Check sheet for the modelled part. Datum: model origin and axes. Units: mm. Round coordinates to 2 decimals unless told otherwise and drop trailing zeros. Write each loop counter-clockwise with the first axis right and the second up, starting at its lowest first coordinate (ties: lowest second). Pieces come first, ordered by that corner, then holes.
Item 1: Section check A-A, the plane x = 104. Record the cut outline in (y, z) (3 decimals), plus the area to 3 significant figures.
Item 2: Material ranges on line 1 along Y through (x, z) = (228.5, 7.25) (3 decimals); line 2 along Z through (x, y) = (-241.3, -2.65), recorded low to high.
Item 3: Release check for a two-part mould opening along Y. For faces 1 (the flat face through (4, 0, 5.556)), 2 (the flat face through (4, -5.556, 0)), 3 (the flat face through (4, 0, -5.556)), 4 (the flat face through (4, 5.556, 0)) record: pulls with the +Y half, pulls with the -Y half, needs draft (parallel to the pull), parting line crosses it, or undercut.
Item 4: Depth check by flat-ended pin: pin 1 (5.5 mm diameter, centred on x = -12.7, y = 0, fed in from +Z); pin 2 (6.5 mm diameter, centred on x = 63.5, z = 0, fed in from +Y). Enter the tip coordinate at first touch or a pass-through.
from build123d import *

# Parameters (mm, degrees)
SKETCH1_W             = 19.05
SKETCH1_H             = 19.05
BOSS_EXTRUDE1_DEPTH   = 254
SKETCH3_W             = 2.4892
SKETCH3_H             = 19.05
SKETCH3_AT_POINT_2_W  = 2.4892
SKETCH3_AT_POINT_2_H  = 19.05
LPATTERN1_START       = -11
LPATTERN1_OUTLINE_R   = 2.4892
LPATTERN1_DEPTH       = 22
LPATTERN1_2_OUTLINE_R = 2.4892
LPATTERN1_2_DEPTH     = 22
SKETCH4_W             = 3.96875
SKETCH4_H             = 7.9375
SKETCH4_W_2           = 7.9375
SKETCH4_H_2           = 3.96875
CUT_EXTRUDE1_DEPTH    = 509.178562368


with BuildPart() as part:
    # Sketch1 → Boss-Extrude1 (new, symmetric)
    with BuildSketch(Plane(origin=(0, 0, 0), x_dir=(0, 0, -1), z_dir=(1, 0, 0))):
        Rectangle(SKETCH1_W, SKETCH1_H)
    extrude(amount=BOSS_EXTRUDE1_DEPTH, both=True)

    # Sketch3 → #9 (0.196) Diameter Hole1 (revolve, cut)
    with BuildSketch(Plane(origin=(241.3, 9.525, 0), x_dir=(0, 0, 1), z_dir=(1, 0, 0))):
        with Locations((1.2446, 9.525)):
            Rectangle(SKETCH3_W, SKETCH3_H)
    revolve(axis=Axis((241.3, 15.875, 0), (0, -1, 0)), mode=Mode.SUBTRACT)

    # Sketch3 at point 2 (carried to point 2, square into its face) → #9 (0.196) Diameter Hole1 at 2 (revolve, cut)
    with BuildSketch(Plane(origin=(241.3, 0, 9.525), x_dir=(0, -1, 0), z_dir=(1, 0, 0))):
        with Locations((1.2446, 9.525)):
            Rectangle(SKETCH3_AT_POINT_2_W, SKETCH3_AT_POINT_2_H)
    revolve(axis=Axis((241.3, 0, 15.875), (0, 0, -1)), mode=Mode.SUBTRACT)

    # LPattern1: read off the stored shape, not the designer's step
    # LPattern1 outline → LPattern1 (cut)
    with BuildSketch(Plane.XY.offset(LPATTERN1_START)):
        with Locations((-241.3, 0)):
            Circle(LPATTERN1_OUTLINE_R)
        with Locations((-215.9, 0)):
            Circle(LPATTERN1_OUTLINE_R)
        with Locations((-190.5, 0)):
            Circle(LPATTERN1_OUTLINE_R)
        with Locations((-165.1, 0)):
            Circle(LPATTERN1_OUTLINE_R)
        with Locations((-139.7, 0)):
            Circle(LPATTERN1_OUTLINE_R)
        with Locations((-114.3, 0)):
            Circle(LPATTERN1_OUTLINE_R)
        with Locations((-88.9, 0)):
            Circle(LPATTERN1_OUTLINE_R)
        with Locations((-63.5, 0)):
            Circle(LPATTERN1_OUTLINE_R)
        with Locations((-38.1, 0)):
            Circle(LPATTERN1_OUTLINE_R)
        with Locations((-12.7, 0)):
            Circle(LPATTERN1_OUTLINE_R)
        with Locations((12.7, 0)):
            Circle(LPATTERN1_OUTLINE_R)
        with Locations((38.1, 0)):
            Circle(LPATTERN1_OUTLINE_R)
        with Locations((63.5, 0)):
            Circle(LPATTERN1_OUTLINE_R)
        with Locations((88.9, 0)):
            Circle(LPATTERN1_OUTLINE_R)
        with Locations((114.3, 0)):
            Circle(LPATTERN1_OUTLINE_R)
        with Locations((139.7, 0)):
            Circle(LPATTERN1_OUTLINE_R)
        with Locations((165.1, 0)):
            Circle(LPATTERN1_OUTLINE_R)
        with Locations((190.5, 0)):
            Circle(LPATTERN1_OUTLINE_R)
        with Locations((215.9, 0)):
            Circle(LPATTERN1_OUTLINE_R)
    extrude(amount=LPATTERN1_DEPTH, mode=Mode.SUBTRACT)

    # LPattern1 2 outline → LPattern1 2 (cut)
    with BuildSketch(Plane(origin=(0, 0, 0), x_dir=(1, 0, 0), z_dir=(0, 1, 0)).offset(LPATTERN1_START)):
        with Locations((215.9, 0)):
            Circle(LPATTERN1_2_OUTLINE_R)
        with Locations((190.5, 0)):
            Circle(LPATTERN1_2_OUTLINE_R)
        with Locations((165.1, 0)):
            Circle(LPATTERN1_2_OUTLINE_R)
        with Locations((139.7, 0)):
            Circle(LPATTERN1_2_OUTLINE_R)
        with Locations((114.3, 0)):
            Circle(LPATTERN1_2_OUTLINE_R)
        with Locations((88.9, 0)):
            Circle(LPATTERN1_2_OUTLINE_R)
        with Locations((63.5, 0)):
            Circle(LPATTERN1_2_OUTLINE_R)
        with Locations((38.1, 0)):
            Circle(LPATTERN1_2_OUTLINE_R)
        with Locations((12.7, 0)):
            Circle(LPATTERN1_2_OUTLINE_R)
        with Locations((-12.7, 0)):
            Circle(LPATTERN1_2_OUTLINE_R)
        with Locations((-38.1, 0)):
            Circle(LPATTERN1_2_OUTLINE_R)
        with Locations((-63.5, 0)):
            Circle(LPATTERN1_2_OUTLINE_R)
        with Locations((-88.9, 0)):
            Circle(LPATTERN1_2_OUTLINE_R)
        with Locations((-114.3, 0)):
            Circle(LPATTERN1_2_OUTLINE_R)
        with Locations((-139.7, 0)):
            Circle(LPATTERN1_2_OUTLINE_R)
        with Locations((-165.1, 0)):
            Circle(LPATTERN1_2_OUTLINE_R)
        with Locations((-190.5, 0)):
            Circle(LPATTERN1_2_OUTLINE_R)
        with Locations((-215.9, 0)):
            Circle(LPATTERN1_2_OUTLINE_R)
        with Locations((-241.3, 0)):
            Circle(LPATTERN1_2_OUTLINE_R)
    extrude(amount=LPATTERN1_2_DEPTH, mode=Mode.SUBTRACT)

    # Sketch4 → Cut-Extrude1 (cut, through all)
    with BuildSketch(Plane(origin=(254, 0, 0), x_dir=(0, 0, -1), z_dir=(1, 0, 0))):
        with Locations((-7.540625, 0)):
            Rectangle(SKETCH4_W, SKETCH4_H)
        with Locations((0, 7.540625)):
            Rectangle(SKETCH4_W_2, SKETCH4_H_2)
        with Locations((7.540625, 0)):
            Rectangle(SKETCH4_W, SKETCH4_H)
        with Locations((0, -7.540625)):
            Rectangle(SKETCH4_W_2, SKETCH4_H_2)
    extrude(amount=-CUT_EXTRUDE1_DEPTH, mode=Mode.SUBTRACT)


solid = part.part
Values found:
1. outline: (-9.525, -9.525) - (-3.969, -9.525) - (-3.969, -5.556) - (3.969, -5.556) - (3.969, -9.525) - (9.525, -9.525) - (9.525, -3.969) - (5.556, -3.969) - (5.556, 3.969) - (9.525, 3.969) - (9.525, 9.525) - (3.969, 9.525) - (3.969, 5.556) - (-3.969, 5.556) - (-3.969, 9.525) - (-9.525, 9.525) - (-9.525, 3.969) - (-5.556, 3.969) - (-5.556, -3.969) - (-9.525, -3.969) - close
1. area: 237 mm2
2. line 1: y = -9.525 to -3.969, 3.969 to 9.525
2. line 2: z = -5.56 to -2.49, 2.49 to 5.56
3. face 1: undercut
3. face 2: pulls with the -Y half
3. face 3: undercut
3. face 4: pulls with the +Y half
4. pin 1: stops at z = 5.56
4. pin 2: stops at y = 5.56
